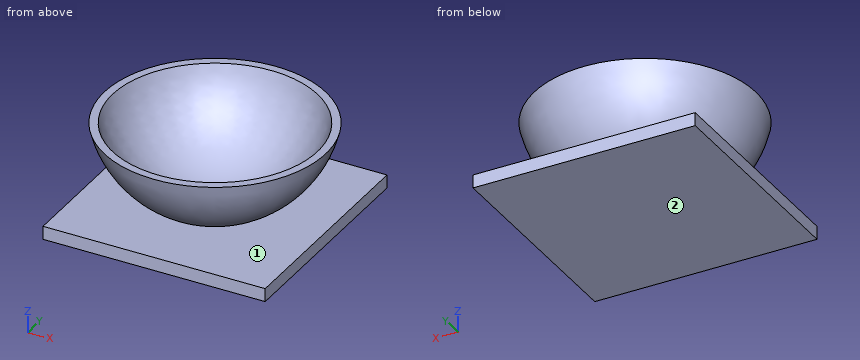
from build123d import *

# Parameters (mm, degrees)
F0_W     = 42
F0_H     = 42
F1_DEPTH = 2.5


with BuildPart() as f1:
    # F0 (on Top) → F1 (new body)
    with BuildSketch(Plane.XY):
        Rectangle(F0_W, F0_H)
    extrude(amount=F1_DEPTH)

    # F2 (on Front) → F3 (revolve)
    with BuildSketch(Plane.XZ):
        with BuildLine():
            ThreePointArc((-20.910524, 17.5), (-13.318221, 5.62176), (0, 1))
            Line((0, 1), (0, 2.5))
            ThreePointArc((0, 2.5), (-12.247449, 6.688612), (-19.364917, 17.5))
            Line((-19.364917, 17.5), (-20.910524, 17.5))
        make_face()
    revolve(axis=Axis((0, 0, 8.75), (0, 0, 1)))


solid = f1.part
Geometry: final body of the model. Coordinates: model frame, mm. Face numbers are marked on the shaded views. Give positions to 0.01 mm unless a question says otherwise; leave off trailing zeros. One line per question, with ' | ' between items. Start each with the question number.
(1) Contact query for flat-ended pins moving along their axis: pin 1 (3 mm diameter, centred on x = 13.5, z = 9, fed in from +Y); pin 2 (10 mm diameter, centred on x = 1, y = -4.5, fed in from +Z); pin 3 (1 mm diameter, centred on x = 3.5, z = 5.5, fed in from -Y). Output: stop coordinate, or through.
(2) Pull-direction query (Z, two-part tool) for the marked faces 1 and 2; classes: released by +Z, released by -Z, zero draft, split by the parting line, or undercut.
(3) Ray query, line 1 (X direction, y = -0.5, z = 7); line 2 (X direction, y = 5, z = 13.5); line 3 (Z direction, x = -8, y = 5). Return the intervals inside material, ascending. Write a range as from..to.
The answers:
1) pin 1: y = 12.36 | pin 2: z = 4.96 | pin 3: y = -13.35
2) face 1: undercut | face 2: released by -Z
3) line 1: -14.89..-12.63, 12.63..14.89 | line 2: -18.87..-17.15, 17.15..18.87 | line 3: 0..2.5, 3.18..4.86
